```python
from build123d import *

# Parameters (mm, degrees)
SKETCH1_R           = 5.5
SKETCH1_R_2         = 1.25
BOSS_EXTRUDE1_DEPTH = 16
BOSS_EXTRUDE2_DEPTH = 1.5
BOSS_EXTRUDE3_DEPTH = 3
CIRPATTERN1_COUNT   = 5
CIRPATTERN1_ANGLE   = 240
FILLET1_R           = 1.5
SKETCH6_R           = 3.5
CUT_EXTRUDE1_DEPTH  = 15.2


with BuildPart() as part:
    # Sketch1 → Boss-Extrude1 (new body)
    with BuildSketch(Plane(origin=(0, 0, 0), x_dir=(1, 0, 0), z_dir=(0, 1, 0))):
        Circle(SKETCH1_R)
        Circle(SKETCH1_R_2, mode=Mode.SUBTRACT)
    extrude(amount=BOSS_EXTRUDE1_DEPTH)

    # Sketch2 → Boss-Extrude2 (add, symmetric)
    with BuildSketch(Plane(origin=(0, 0, 0), x_dir=(0, 0, -1), z_dir=(1, 0, 0))):
        with BuildLine():
            Line((18, -5), (20, -5))
            add(Edge.make_bspline(
                [(8.914213562, 14.585786438), (13.074333826, 10.425666174), (20, 1.461761402), (20, -5)],
                knots=[0.14734609, 0.14734609, 0.14734609, 0.14734609, 1, 1, 1, 1], degree=3))
            Line((8.914213562, 14.585786438), (7.5, 16))
            Line((7.5, 16), (5.5, 16))
            Line((5.5, 16), (1.25, 16))
            Line((1.25, 16), (1.25, 4))
            Line((1.25, 4), (6.70571865, 4))
            add(Edge.make_bspline(
                [(6.70571865, 4), (10.522194615, 4), (16.021169224, 3.257262603), (18, -4.005650027), (18, -5)],
                knots=[0, 0, 0, 0, 0.785490543, 1, 1, 1, 1], degree=3))
        make_face()
    boss_extrude2 = extrude(amount=BOSS_EXTRUDE2_DEPTH, both=True)

    # Sketch8 → Boss-Extrude3 (add)
    with BuildSketch(Plane(origin=(1.5, 0, 0), x_dir=(0, 0, -1), z_dir=(1, 0, 0))):
        Polygon((18, -7), (17.788407623, -8.2), (17.894203812, -9.409255967), (19.894203812, -9.409255967), (20, -8.2), (20, -7), (20, -5), (18, -5), align=None)
    boss_extrude3 = extrude(amount=-BOSS_EXTRUDE3_DEPTH)

    # CirPattern1: Boss-Extrude2, Boss-Extrude3 ×5 about axis
    cirpattern1_axis = Axis((0, 16, 0), (0, -1, 0))
    for i in range(1, CIRPATTERN1_COUNT):
        add(boss_extrude2.rotate(cirpattern1_axis, i * CIRPATTERN1_ANGLE / (CIRPATTERN1_COUNT - 1)))
        add(boss_extrude3.rotate(cirpattern1_axis, i * CIRPATTERN1_ANGLE / (CIRPATTERN1_COUNT - 1)))

    # Fillet1
    fillet1_edges = [part.edges().sort_by_distance(p)[0] for p in [
        (-5.332575695, 10, 1.346713205),
        (1.5, 10, -5.291502622),
        (-1.5, 10, -5.291502622),
        (3.832575695, 10, -3.944789417),
        (5.332575695, 10, 1.346713205),
        (1.5, 10, 5.291502622),
        (-3.832575695, 10, 3.944789417),
        (5.332575695, 10, -1.346713205),
        (3.832575695, 10, 3.944789417),
        (-1.5, 10, 5.291502622),
    ]]
    fillet(fillet1_edges, radius=FILLET1_R)

    # Sketch6 → Cut-Extrude1 (cut)
    with BuildSketch(Plane(origin=(0, 16, 0), x_dir=(1, 0, 0), z_dir=(0, 1, 0))):
        Circle(SKETCH6_R)
    extrude(amount=-CUT_EXTRUDE1_DEPTH, mode=Mode.SUBTRACT)


solid = part.part
```
For this review, take the finished solid that the model builds, in its own axes (mm). A direction names the side the tool comes from. Round coordinates to 2 decimals unless told otherwise and drop trailing zeros. Write each loop counter-clockwise with the first axis right and the second up, starting at its lowest first coordinate (ties: lowest second). Pieces come first, ordered by that corner, then holes. Notation, with made-up numbers: (-37, 73.25) -> (-19, 73.25) arc R12 ccw to (-19, 79.25) -> close; hole circle Ø11 at (39, -10). An arc over 180 degrees is marked (long way). One line per question, with ' | ' between items. Start each with the question number.
1) For pin 1 Ø0.5 at (x, z) = (-0.5, 6) entering from -Y; pin 2 Ø11 at (y, z) = (3, 14) entering from -X; pin 3 Ø12 at (y, z) = (8, -16) entering from -X; pin 4 Ø11 at (x, z) = (0, 0) entering from +Y, all flat-tipped, find the tip position at first contact; note any pin that passes through.
2) Add section A-A (y = -7.5). Write out the cut boundary in (x, z).
3) Add section C-C (y = -0.75). Count the separate pieces of the cut face and the enclosed holes in it, and give its area (3 significant figures).
4) Machinability: for faces 1 (the flat face through (-0.02, -8.8, 17.84)), 2 (the flat face through (0.021, -7.592, -17.896)), 3 (the flat face through (9.744, 5.237, 7.358)), which of the approach directions +Z, -Z, +X, -X, +Y, -Y give a long, thin tool a straight path to every point of the face, cutting with its end or side? Answer none if there is none.
5) Add section B-B (x = 4). Write out the cut boundary in (y, z), and give its area (3 significant figures).
6) Wall thickness on line 1 along X through (y, z) = (0.4, 0); line 2 along X through (y, z) = (5.25, 0); line 3 along Z through (x, y) = (0.5, -5.75): over which ranges is each line inside the solid? List them lowest first.
7) Mouldability with a two-part tool opening along Y and no side actions: class faces 4 (the flat face through (0, -6, -18)), 5 (the cylindrical face through (-1.74, 9.92, 5.51)), 6 (the flat face through (-17.285, -8.813, 9.955)) as +Y half, -Y half, draft (parallel to the pull), parting line (faces both ways), or undercut.
Reported:
1) pin 1: stops at y = 4 | pin 2: stops at x = -16.45 | pin 3: stops at x = -1.5 | pin 4: stops at y = 16
2) outline: (-18.07, 8.7) -> (-16.26, 7.66) -> (-14.76, 10.25) -> (-16.57, 11.3) -> close; (-1.5, -20) -> (1.5, -20) -> (1.5, -17.91) -> (-1.5, -17.91) -> close; (-1.5, 17.91) -> (1.5, 17.91) -> (1.5, 20) -> (-1.5, 20) -> close; (14.76, -10.25) -> (16.57, -11.3) -> (18.07, -8.7) -> (16.26, -7.66) -> close; (14.76, 10.25) -> (16.26, 7.66) -> (18.07, 8.7) -> (16.57, 11.3) -> close
3) separate pieces: 5 | enclosed holes: 0 | area: 36.5 mm²
4) face 1: +X, -X, -Y | face 2: +X, -X | face 3: +Z, +Y, -Y
5) outline: (0, -3.77) -> (4, -3.77) -> (4, -4.26) -> (16, -4.26) -> (16, 4.26) -> (4, 4.26) -> (4, 3.77) -> (0, 3.77) -> close | area: 132 mm²
6) line 1: x = -5.5 to -1.25, 1.25 to 5.5 | line 2: x = -5.5 to -3.5, 3.5 to 5.5 | line 3: z = -20 to -18, 18 to 20
7) face 4: undercut | face 5: draft | face 6: -Y half
